from build123d import *

# Parameters (mm, degrees)
F0_W          = 300
F0_H          = 160
F1_DEPTH      = 40
F4_W          = 45
F4_H          = 160
F3_W          = 45
F3_H          = 160
F7_W          = 25.3585465252
F7_H          = 50.359621644
F8_DEPTH      = 144.1733793765
F8_DEPTH_BACK = 144.1733793765


with BuildPart() as f1:
    # F0 (on Top) → F1 (new body)
    with BuildSketch(Plane.XY):
        Rectangle(F0_W, F0_H)
    extrude(amount=F1_DEPTH)

    # F6: F5 across plane


with BuildPart() as f5:
    # F4 (on face) → F5 section 0
    with BuildSketch(Plane(origin=(0, 0, 0), x_dir=(1, 0, 0), z_dir=(0, 0, -1))):
        with Locations((127.5, 0)):
            Rectangle(F4_W, F4_H)
    # F3 (on offset) → F5 section 1
    with BuildSketch(Plane(origin=(0, 0, -180), x_dir=(1, 0, 0), z_dir=(0, 0, -1))):
        with Locations((172.5, 0)):
            Rectangle(F3_W, F3_H)
    loft()


with BuildPart() as f1_1:
    add(f1.part)
    add(f5.part.mirror(Plane.YZ))


    add(f5.part)  # F8 merges F5
    # F7 (on Right) → F8 (join, two sides)
    with BuildSketch(Plane.YZ) as f8_sk:
        with Locations((0, -127.5137066841)):
            Rectangle(F7_W, F7_H)
    extrude(amount=F8_DEPTH)
    extrude(f8_sk.sketch, amount=-F8_DEPTH_BACK)


solid = f1_1.part
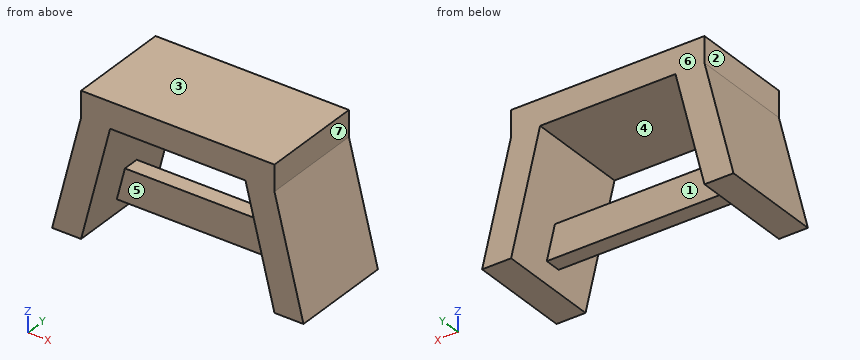
Here's how the part is built. I have some questions about the finished solid (model axes, mm). Face numbers are marked on the shaded views. A direction names the side the tool comes from. Coordinates: 2 decimals unless noted, no trailing zeros. Loops run counter-clockwise (first coordinate to the right, second up) from the corner with the lowest first, then second, coordinate; pieces in that order, holes last. Notation, with made-up numbers: (-37, 15) -> (2, 15) arc R25 cw to (2, 41) -> close; hole circle Ø6 at (45.25, -12). An arc over 180 degrees is marked (long way). Use one line per item in the form item = value. Start each with the question number.
(1) If we section it at A-A (x = 45.5): Please give me the cut outline in (y, z), then the cut area to 3 significant figures.
(2) Will these pins go through, and if not, where does the flat tip stop? pin 1 (25 mm diameter, centred on x = -11, z = -125, fed in from -Y); pin 2 (12 mm diameter, centred on y = 59.5, z = -7.5, fed in from +X) (3 decimals); pin 3 (2 mm diameter, centred on y = -16.5, z = -151.5, fed in from +X) (3 decimals).
(3) Please list where these lines run through material, in increasing order: line 1 along X through (y, z) = (37, 4); line 2 along Z through (x, y) = (-20.5, -23); line 3 along Z through (x, y) = (49.5, -3).
(4) If we section it at B-B (z = -40): Please give me the cut outline in (x, y).
(5) If we section it at D-D (x = 138): Please give me the cut outline in (y, z), then the cut area to 3 significant figures.
(6) If we section it at C-C (y = 69.5): Please give me the cut outline in (x, z), then the cut area to 3 significant figures.
(7) On a 3-axis mill with a long thin cutter (end or side, diameter ignored), from which of +Z, -Z, +X, -X, +Y, -Y can I reach the whole of each face in a straight line? I mean the marked faces 5, 6 and 7. Say none if no direction works.
(8) We'd pull the mould along X, two halves only. Please class the marked faces 1, 2, 3 and 4: pulls with the +X half, pulls with the -X half, needs draft (parallel to the pull), parting line crosses it, or undercut.
Verdict:
q1.outline = (-80, 0) -> (80, 0) -> (80, 40) -> (-80, 40) -> close; (-12.68, -152.69) -> (12.68, -152.69) -> (12.68, -102.33) -> (-12.68, -102.33) -> close
q1.area = 7,680 mm²
q2.pin_1 = -12.68
q2.pin_2 = 153.375
q2.pin_3 = 188.125
q3.line_1 = -150 to 150
q3.line_2 = 0 to 40
q3.line_3 = -152.69 to -102.33, 0 to 40
q4.outline = (-160, -80) -> (-115, -80) -> (-115, 80) -> (-160, 80) -> close; (115, -80) -> (160, -80) -> (160, 80) -> (115, 80) -> close
q5.outline = (-80, -132) -> (-12.68, -132) -> (-12.68, -152.69) -> (12.68, -152.69) -> (12.68, -132) -> (80, -132) -> (80, 40) -> (-80, 40) -> close
q5.area = 28,000 mm²
q6.outline = (-195, -180) -> (-150, -180) -> (-105, 0) -> (105, 0) -> (150, -180) -> (195, -180) -> (150, 0) -> (150, 40) -> (-150, 40) -> (-150, 0) -> close
q6.area = 28,200 mm²
q7.face_5 = -Z, -Y
q7.face_6 = +Z, -Z, +X, -X, +Y
q7.face_7 = +Z, +X, +Y, -Y
q8.face_1 = undercut
q8.face_2 = pulls with the -X half
q8.face_3 = needs draft
q8.face_4 = undercut
